Could you check a few things on this model? Use its own coordinates, in mm. A direction names the side the tool comes from. Coordinates: 2 decimals unless noted, no trailing zeros. Loops run counter-clockwise (first coordinate to the right, second up) from the corner with the lowest first, then second, coordinate; pieces in that order, holes last.
from build123d import *

# Parameters (mm, degrees)
SKETCH1_R               = 37.5
BOSS_EXTRUDE1_DEPTH     = 579.5
SKETCH2_R               = 75
BOSS_EXTRUDE2_DEPTH     = 200
CUT_EXTRUDE1_DEPTH      = 787.683068332
CUT_EXTRUDE1_DEPTH_BACK = 787.683068332
SKETCH3_R               = 25
CUT_EXTRUDE2_DEPTH      = 795.691831969
CUT_EXTRUDE2_DEPTH_BACK = 795.691831969
SKETCH5_W               = 222.214700053
SKETCH5_H               = 39.823422949


with BuildPart() as part:
    # Sketch1 → Boss-Extrude1 (new, symmetric)
    with BuildSketch(Plane.XY):
        Circle(SKETCH1_R)
    extrude(amount=BOSS_EXTRUDE1_DEPTH, both=True)

    # Sketch2 → Boss-Extrude2 (add)
    with BuildSketch(Plane(origin=(0, 0, -579.5), x_dir=(-1, 0, 0), z_dir=(0, 0, -1))):
        Circle(SKETCH2_R)
    extrude(amount=BOSS_EXTRUDE2_DEPTH)

    # Sketch3 → Cut-Extrude1 (cut, two sides: drawn at the far end of the back side and taken through both)
    with BuildSketch(Plane(origin=(0, 0, 0), x_dir=(1, 0, 0), z_dir=(0, 1, 0)).offset(-CUT_EXTRUDE1_DEPTH_BACK)):
        with Locations(Location((0, 719.26, 0), (0, 0, 270))):
            Circle(SKETCH3_R)
        with BuildLine():
            Line((75, 579.5), (60.24, 646.55))
            Line((60.24, 646.55), (60.24, 719.26))
            ThreePointArc((60.24, 719.26), (0, 779.5), (-60.24, 719.26))
            Line((-60.24, 719.26), (-60.24, 646.55))
            Line((-60.24, 646.55), (-75, 579.5))
            Line((-75, 579.5), (-116.955269632, 579.5))
            Line((-116.955269632, 579.5), (-116.955269632, 829.791162558))
            Line((-116.955269632, 829.791162558), (115.893588729, 829.791162558))
            Line((115.893588729, 829.791162558), (115.893588729, 579.5))
            Line((115.893588729, 579.5), (75, 579.5))
        make_face()
    extrude(amount=CUT_EXTRUDE1_DEPTH + CUT_EXTRUDE1_DEPTH_BACK, mode=Mode.SUBTRACT)

    # Sketch5 → Cut-Extrude2 (cut, two sides: drawn at the far end of the back side and taken through both)
    with BuildSketch(Plane.ZY.offset(60.24).offset(-CUT_EXTRUDE2_DEPTH_BACK)):
        with Locations((-711.467350027, 82.581711474)):
            Rectangle(SKETCH5_W, SKETCH5_H)
        with Locations((-711.467350027, -82.581711474)):
            Rectangle(SKETCH5_W, SKETCH5_H)
    extrude(amount=CUT_EXTRUDE2_DEPTH + CUT_EXTRUDE2_DEPTH_BACK, mode=Mode.SUBTRACT)


solid = part.part
1) We'd pull the mould along Z, two halves only. Please class faces 1 (the cylindrical face through (1.099, -0.877, -744.236)), 2 (the flat face through (-15.6, 34.4, -579.5)), 3 (the flat face through (66.083, -0.625, -620.006)), 4 (the flat face through (60.24, -1, -682)): released by +Z, released by -Z, zero draft, split by the parting line, or undercut.
2) For faces 5 (the flat face through (1, 62.67, -691)), 6 (the flat face through (-60.24, -1, -683)), 7 (the cylindrical face through (-4.88, 37.18, 8.11)), 8 (the flat face through (1, -62.67, -691)), which set-ups out of +Z, -Z, +X, -X, +Y, -Y let a thin tool reach every point of the face, with its end or its side?
3) Imagine slicing it at C-C on z = 275.5. List the corners of the cut face in (x, y) for me.
4) If I drill on L1, parallel to X at y = 4, z = -719.26; L2, parallel to Z at x = 0, y = -10; L3, parallel to Y at x = 1, z = 366.5, over which ranges is the centre line in solid material (lowest first)?
5) Will these pins go through, and if not, where does the flat tip stop? pin 1 (24.5 mm diameter, centred on x = 17, z = -662, fed in from -Y); pin 2 (12 mm diameter, centred on x = -39.5, y = -56.5, fed in from +Z); pin 3 (1 mm diameter, centred on x = 41.5, y = 60, fed in from -Z).
6) Imagine slicing it at B-B on y = 13.5. List the corners of the cut face in (x, z) for me (3 decimals), plus the area to 3 significant figures.
7) Imagine slicing it at A-A on x = 0. List the corners of the cut face in (y, z) for me.
Solved:
1. face 1: undercut
1. face 2: released by +Z
1. face 3: released by -Z
1. face 4: zero draft
2. face 5: -Z, +X, -X, +Y
2. face 6: -Z, -X, +Y, -Y
2. face 7: +Z
2. face 8: -Z, +X, -X, -Y
3. outline: circle Ø75 at (0, 0)
4. L1: x = -60.24 to -25, 25 to 60.24
4. L2: z = -779.5 to -744.26, -694.26 to 579.5
4. L3: y = -37.49 to 37.49
5. pin 1: stops at y = -62.67
5. pin 2: stops at z = -579.5
5. pin 3: stops at z = -763.39
6. outline: (-73.775, -585.065) - (-60.24, -646.55) - (-60.24, -719.26) arc R60.24 ccw to (60.24, -719.26) - (60.24, -646.55) - (73.775, -585.065) - (73.775, -579.5) - (34.986, -579.5) - (34.986, 579.5) - (-34.986, 579.5) - (-34.986, -579.5) - (-73.775, -579.5) - close; hole circle Ø50 at (0, -719.26)
6. area: 103,000 mm2
7. outline: (-75, -600.36) - (-62.67, -600.36) - (-62.67, -694.26) - (62.67, -694.26) - (62.67, -600.36) - (75, -600.36) - (75, -579.5) - (37.5, -579.5) - (37.5, 579.5) - (-37.5, 579.5) - (-37.5, -579.5) - (-75, -579.5) - close; (-62.67, -779.5) - (62.67, -779.5) - (62.67, -744.26) - (-62.67, -744.26) - close
